Can you work these out from the model? Positions are in its coordinate system, mm. Give positions to 0.01 mm unless a question says otherwise; leave off trailing zeros. Write each loop counter-clockwise with the first axis right and the second up, starting at its lowest first coordinate (ties: lowest second). Pieces come first, ordered by that corner, then holes. Notation, with made-up numbers: (53.5, 62.25) -> (88.5, 62.25) arc R25 cw to (88.5, 81.25) -> close; hole circle Ø11 at (-13, 31). An arc over 180 degrees is marked (long way). One line per item, written item: value.
from build123d import *

# Parameters (mm, degrees)
F1_DEPTH = 12.954
F2_R     = 10.50497
F3_DEPTH = 10.668


with BuildPart() as f1:
    # F0 (on Front) → F1 (new body)
    with BuildSketch(Plane.XZ):
        Polygon((22.575585, 17.971164), (-35.091735, 32.122731), (-39.053906, 5.805923), (-8.221038, 2.165531), (-4.384858, -32.257307), (40.195391, -27.289156), align=None)
    extrude(amount=-F1_DEPTH)

    # F2 (on face) → F3 (join)
    with BuildSketch(Plane(origin=(0, 12.954, 0), x_dir=(-1, 0, 0), z_dir=(0, 1, 0))):
        with Locations((-14.078603, 2.165531)):
            Circle(F2_R)
    extrude(amount=-F3_DEPTH)


solid = f1.part
1) If we section it at A-A (y = 4.5): Write out the boundary of the cut face in (x, z), and give its area (3 significant figures).
Answer list:
outline: (-39.05, 5.81) -> (-8.22, 2.17) -> (-4.38, -32.26) -> (40.2, -27.29) -> (22.58, 17.97) -> (-35.09, 32.12) -> close
area: 2,700 mm^2
2) If we section it at B-B (z = -5): Write out the boundary of the cut face in (x, y), and give its area (3 significant figures).
Answer list:
outline: (-7.42, 0) -> (31.52, 0) -> (31.52, 12.95) -> (-7.42, 12.95) -> close
area: 504 mm^2
3) Will these pins go through, and if not, where does the flat tip stop? pin 1 (1 mm diameter, centred on y = 2.5, z = -10.5, fed in from +X); pin 2 (5 mm diameter, centred on y = 6, z = -14.5, fed in from -X).
Answer list:
pin 1: stops at x = 33.85
pin 2: stops at x = -6.64
4) I need wall thicknesses on L1, parallel to X at y = 8.25, z = -12; L2, parallel to X at y = 7, z = -21.5; L3, parallel to Z at x = -3, y = 3. Which ranges of each line are inside material? Lowest first, please.
Answer list:
L1: x = -6.64 to 34.24
L2: x = -5.58 to 37.94
L3: z = -32.1 to 24.25
5) If we section it at C-C (x = -12): Write out the boundary of the cut face in (y, z), and give its area (3 significant figures).
Answer list:
outline: (0, 2.61) -> (12.95, 2.61) -> (12.95, 26.46) -> (0, 26.46) -> close
area: 309 mm^2
